from build123d import *

# Parameters (mm, degrees)
SKETCH_1_W          = 588
SKETCH_1_H          = 490
EXTRUDE_1_DEPTH     = 154
SKETCH_2_R          = 80
CUT_EXTRUDE_1_DEPTH = 45
SKETCH_3_W          = 155
SKETCH_3_H          = 105
SKETCH_3_W_2        = 105
SKETCH_3_H_2        = 155
SKETCH_3_W_3        = 135
CUT_EXTRUDE_2_DEPTH = 99
CHAMFER_1_SIZE      = 80
SKETCH_4_W          = 45
SKETCH_4_H          = 155
SKETCH_4_W_2        = 155
SKETCH_4_H_2        = 45
SKETCH_4_W_3        = 50
CUT_EXTRUDE_3_DEPTH = 56
CHAMFER_2_SIZE      = 20
CHAMFER_3_SIZE      = 35
SKETCH_5_W          = 85
SKETCH_5_H          = 155
CUT_EXTRUDE_4_DEPTH = 47
SKETCH_6_R          = 12.5
CUT_EXTRUDE_5_DEPTH = 10
CHAMFER_4_SIZE      = 10
SKETCH_7_W          = 28.842878722
SKETCH_7_H          = 45
CUT_EXTRUDE_6_DEPTH = 155
CHAMFER_6_SIZE      = 10
CUT_EXTRUDE_7_DEPTH = 45
CUT_EXTRUDE_START   = -490
CUT_EXTRUDE_8_DEPTH = 45
SKETCH_9_W          = 45
SKETCH_9_H          = 60
CUT_EXTRUDE_9_DEPTH = 50
CHAMFER_7_SIZE      = 20


with BuildPart() as part:
    # 草图1 → 凸台-拉伸1 (new body)
    with BuildSketch(Plane(origin=(0, 0, 0), x_dir=(1, 0, 0), z_dir=(0, 1, 0))):
        Rectangle(SKETCH_1_W, SKETCH_1_H)
    extrude(amount=EXTRUDE_1_DEPTH)

    # 草图2 → 切除-拉伸1 (cut)
    with BuildSketch(Plane.XY.offset(245)):
        with Locations((-196.5, 26)):
            Circle(SKETCH_2_R)
        with Locations((189.5, 26)):
            Circle(SKETCH_2_R)
    cut_extrude_1 = extrude(amount=-CUT_EXTRUDE_1_DEPTH, mode=Mode.SUBTRACT)

    # 镜向1: 切除-拉伸1 across plane
    add(cut_extrude_1.mirror(Plane.XY), mode=Mode.SUBTRACT)

    # 草图3 → 切除-拉伸2 (cut)
    with BuildSketch(Plane(origin=(0, 154, 0), x_dir=(1, 0, 0), z_dir=(0, 1, 0))):
        with Locations((0, -192.5)):
            Rectangle(SKETCH_3_W, SKETCH_3_H)
        with Locations((241.5, 0)):
            Rectangle(SKETCH_3_W_2, SKETCH_3_H_2)
        with Locations((0, 192.5)):
            Rectangle(SKETCH_3_W, SKETCH_3_H)
        with Locations((-226.5, 0)):
            Rectangle(SKETCH_3_W_3, SKETCH_3_H_2)
    extrude(amount=-CUT_EXTRUDE_2_DEPTH, mode=Mode.SUBTRACT)

    # 倒角1
    chamfer_1_edges = [part.edges().sort_by_distance(p)[0] for p in [
        (294, 154, 161.25),
        (294, 154, -161.25),
    ]]
    chamfer(chamfer_1_edges, length=CHAMFER_1_SIZE)

    # 草图4 → 切除-拉伸3 (cut, through all)
    with BuildSketch(Plane(origin=(0, 55, 0), x_dir=(1, 0, 0), z_dir=(0, 1, 0))):
        with Locations((271.5, 0)):
            Rectangle(SKETCH_4_W, SKETCH_4_H)
        with Locations((0, 222.5)):
            Rectangle(SKETCH_4_W_2, SKETCH_4_H_2)
        with Locations((0, -222.5)):
            Rectangle(SKETCH_4_W_2, SKETCH_4_H_2)
        with Locations((-269, 0)):
            Rectangle(SKETCH_4_W_3, SKETCH_4_H)
    extrude(amount=-CUT_EXTRUDE_3_DEPTH, mode=Mode.SUBTRACT)

    # 倒角2
    chamfer_2_edges = [part.edges().sort_by_distance(p)[0] for p in [
        (294, 37, -77.5),
        (294, 37, 77.5),
        (77.5, 77, -245),
        (-77.5, 77, -245),
        (77.5, 77, 245),
        (-77.5, 77, 245),
        (-294, 77, 77.5),
        (-294, 77, -77.5),
    ]]
    chamfer(chamfer_2_edges, length=CHAMFER_2_SIZE)

    # 倒角3
    chamfer_3_edges = [part.edges().sort_by_distance(p)[0] for p in [
        (-294, 154, 171.25),
        (-294, 154, -171.25),
    ]]
    chamfer(chamfer_3_edges, length=CHAMFER_3_SIZE)

    # 草图5 → 切除-拉伸4 (cut)
    with BuildSketch(Plane(origin=(0, 55, 0), x_dir=(1, 0, 0), z_dir=(0, 1, 0))):
        with Locations((-201.5, 0)):
            Rectangle(SKETCH_5_W, SKETCH_5_H)
    extrude(amount=-CUT_EXTRUDE_4_DEPTH, mode=Mode.SUBTRACT)

    # 草图6 → 切除-拉伸5 (cut)
    with BuildSketch(Plane(origin=(0, 154, 0), x_dir=(1, 0, 0), z_dir=(0, 1, 0))):
        with Locations((-3.5, 0)):
            Circle(SKETCH_6_R)
    extrude(amount=-CUT_EXTRUDE_5_DEPTH, mode=Mode.SUBTRACT)

    # 倒角4
    chamfer_4_edges = [part.edges().sort_by_distance(p)[0] for p in [
        (-294, 59.5, 245),
        (-294, 59.5, -245),
    ]]
    chamfer(chamfer_4_edges, length=CHAMFER_4_SIZE)

    # 草图7 → 切除-拉伸6 (cut, through all)
    with BuildSketch(Plane.XZ):
        with Locations((279.578560639, 222.5)):
            Rectangle(SKETCH_7_W, SKETCH_7_H)
        with Locations((279.578560639, -222.5)):
            Rectangle(SKETCH_7_W, SKETCH_7_H)
    extrude(amount=-CUT_EXTRUDE_6_DEPTH, mode=Mode.SUBTRACT)

    # 倒角6
    chamfer_6_edges = [part.edges().sort_by_distance(p)[0] for p in [
        (294, 37, 200),
        (294, 37, -200),
    ]]
    chamfer(chamfer_6_edges, length=CHAMFER_6_SIZE)

    # 草图8 → 切除-拉伸7 (cut)
    with BuildSketch(Plane.XY.offset(245)):
        with BuildLine():
            Line((265.157121278, 77.421439361), (250.78487231, 77.421439361))
            ThreePointArc((250.78487231, 77.421439361), (259.140791184, 65.372073901), (265.157121278, 52))
            Line((265.157121278, 52), (265.157121278, 77.421439361))
        make_face()
    extrude(amount=-CUT_EXTRUDE_7_DEPTH, mode=Mode.SUBTRACT)

    # 草图8<2> → 切除-拉伸8 (cut)
    with BuildSketch(Plane.XY.offset(245).offset(CUT_EXTRUDE_START)):
        with BuildLine():
            Line((265.157121278, 77.421439361), (250.78487231, 77.421439361))
            ThreePointArc((250.78487231, 77.421439361), (259.140791184, 65.372073901), (265.157121278, 52))
            Line((265.157121278, 52), (265.157121278, 77.421439361))
        make_face()
    extrude(amount=CUT_EXTRUDE_8_DEPTH, mode=Mode.SUBTRACT)

    # 草图9 → 切除-拉伸9 (cut)
    with BuildSketch(Plane.ZY.offset(294)):
        with Locations((222.5, 30)):
            Rectangle(SKETCH_9_W, SKETCH_9_H)
        with Locations((-222.5, 30)):
            Rectangle(SKETCH_9_W, SKETCH_9_H)
    extrude(amount=-CUT_EXTRUDE_9_DEPTH, mode=Mode.SUBTRACT)

    # 倒角7
    chamfer_7_edges = [part.edges().sort_by_distance(p)[0] for p in [
        (-294, 0, -148.75),
        (-294, 0, 148.75),
        (294, 0, -143.75),
        (294, 0, 143.75),
    ]]
    chamfer(chamfer_7_edges, length=CHAMFER_7_SIZE)


solid = part.part
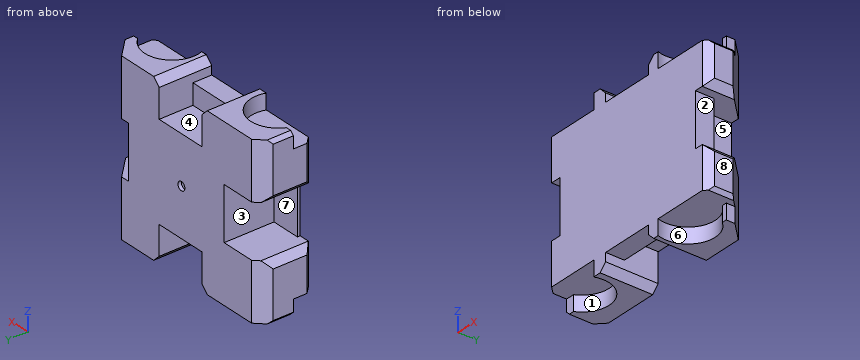
The listing builds one solid part. Answer for the finished solid, in the listing's coordinates (mm). Face numbers are marked on the shaded views. A direction names the side the tool comes from. Give positions to 0.01 mm unless a question says otherwise; leave off trailing zeros. Write each loop counter-clockwise with the first axis right and the second up, starting at its lowest first coordinate (ties: lowest second). Pieces come first, ordered by that corner, then holes. Notation, with made-up numbers: (-34, -18.75) - (13, -18.75) arc R11 ccw to (13, -6.75) - close; hole circle Ø10 at (3, -2.75). An arc over 180 degrees is marked (long way). One line per question, with ' | ' between items. Start each with the question number.
1. For the marked faces 1, 2, 3, 4 and 5, determine the directions among +Z, -Z, +X, -X, +Y, -Y from which every point of the face is accessible in a straight line to the end or side of a thin tool.
2. Section B-B, the plane x = -196.5 is taken. Determine the outline of the cut face in (y, z).
3. Determine the mould class of the marked faces 6, 7 and 8 for opening direction Y: +Y half, -Y half, draft (parallel to the pull), parting line (faces both ways), or undercut.
4. Straight lines are drawn through the part: line 1 (X direction, y = 147.25, z = 0); line 2 (Z direction, x = -3.5, y = 151.25); line 3 (Z direction, x = -250.5, y = 64). For each, find the intervals that lie inside material, in ascending order.
5. Section C-C, the plane z = 214 is taken. Determine the outline of the cut face in (x, y).
6. Section A-A, the plane z = 28 is taken. Determine the outline of the cut face in (x, y), then the cut area to 3 significant figures.
7. Section D-D, the plane x = -3.5 is taken. Determine the outline of the cut face in (y, z).
8. Given P1, Ø20, axis at x = -287, z = -214, coming from the -Y side; P2, Ø10, axis at y = 138, z = -34, coming from the +X side; P3, Ø1, axis at x = 234.5, z = 33.5, coming from the +Y side, each flat-ended and moving along its own axis, determine where each tip first touches the part or whether it passes through.
Result:
1) face 1: -Z | face 2: +X, +Y, -Y | face 3: -X, +Y | face 4: +Z, +Y | face 5: +X, +Y
2) outline: (0, -200) - (106, -200) - (106, -245) - (154, -245) - (154, -77.5) - (8, -77.5) - (8, 77.5) - (154, 77.5) - (154, 245) - (106, 245) - (106, 200) - (0, 200) - close
3) face 6: undercut | face 7: +Y half | face 8: draft
4) line 1: x = -159 to -16, 9 to 189 | line 2: z = -140 to -12.5, 12.5 to 140 | line 3: z = -200 to -77.5, 77.5 to 200
5) outline: (-294, 60) - (-268.92, 60) arc R80 cw to (-120.84, 0) - (-77.5, 0) - (-77.5, 154) - (-259, 154) - (-294, 119) - close; (77.5, 0) - (113.84, 0) arc R80 cw to (250.78, 77.42) - (265.16, 77.42) - (265.16, 102.84) - (214, 154) - (77.5, 154) - close
6) outline: (-244, 0) - (249, 0) - (249, 55) - (189, 55) - (189, 154) - (-159, 154) - (-159, 8) - (-244, 8) - close | area: 57,600 mm2
7) outline: (0, -200) - (55, -200) - (55, -140) - (154, -140) - (154, -12.5) - (144, -12.5) - (144, 12.5) - (154, 12.5) - (154, 140) - (55, 140) - (55, 200) - (0, 200) - close
8) P1: stops at y = 60 | P2: stops at x = 189 | P3: stops at y = 55
